Work out the finished part from the listing and answer in its coordinate system (mm). Round coordinates to 2 decimals unless told otherwise and drop trailing zeros. Order: outer loops, then holes, each group sorted by start corner. A loop starts at its lowest first (then second) coordinate and runs counter-clockwise, first axis right, second up.
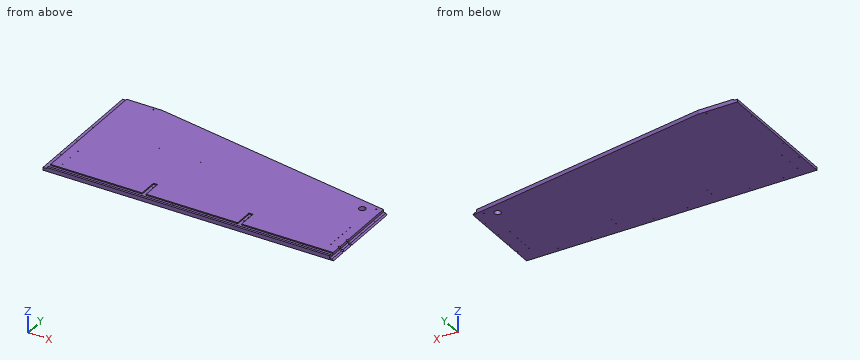
from build123d import *

# Parameters (mm, degrees)
CABSIDERIGHT_THICKNESS_DEPTH  = 17.78
LEDGECUTS_DEPTH_DEPTH         = 5.08
SKETCH9_R                     = 3.301999998
SKETCH9_R_2                   = 3.174999998
SKETCH9_R_3                   = 3.174999999
CUT_EXTRUDE4_DEPTH            = 5.08
SKETCH10_R                    = 15.08125
SKETCH10_R_2                  = 1.5875
CUT_EXTRUDE5_DEPTH            = 17.78
FRONTLEDGECUT_W               = 17.78
FRONTLEDGECUT_H               = 402.324113577
FRONTLEDGECUT_THICKNESS_DEPTH = 11.43
CUT_EXTRUDE8_DEPTH            = 594.36
SKETCH15_R                    = 2.38125
CUT_EXTRUDE9_DEPTH            = 17.78
SKETCH16_R                    = 1.5875
CUT_EXTRUDE10_DEPTH           = 12.7
SKETCH17_R                    = 4.7625
CUT_EXTRUDE11_DEPTH           = 76.2


with BuildPart() as part:
    # CabSideRight_Outline → CabSideRight_Thickness (new body)
    with BuildSketch(Plane.XY):
        Polygon((9092.234544556, -4658.6775), (10222.970833334, -4853.78125), (10222.970833334, -5253.0375), (8914.870833334, -5253.0375), (8914.870833334, -4658.6775), align=None)
    extrude(amount=-CABSIDERIGHT_THICKNESS_DEPTH)

    # CabSideRight_LedgeCuts → LedgeCuts_Depth (cut)
    with BuildSketch(Plane.XY):
        Polygon((8932.650833334, -4658.6775), (8914.870833334, -4658.6775), (8914.870833334, -5253.0375), (8932.650833334, -5253.0375), (8932.650833334, -5243.5125), (10222.970833334, -5243.5125), (10222.970833334, -5225.7325), (9792.864166668, -5225.7325), (9792.864166668, -5141.912499999), (9775.084166668, -5141.912499999), (9775.084166668, -5225.7325), (9362.757500002, -5225.7325), (9362.757500002, -5141.9125), (9344.977500002, -5141.912499999), (9344.977500002, -5225.7325), (8932.650833334, -5225.7325), align=None)
    extrude(amount=-LEDGECUTS_DEPTH_DEPTH, mode=Mode.SUBTRACT)

    # Sketch9 → Cut-Extrude4 (cut)
    with BuildSketch(Plane.XY):
        with Locations((9347.222564031, -5144.157564028)):
            Circle(SKETCH9_R)
        with Locations((9360.512435973, -5144.15756403)):
            Circle(SKETCH9_R_2)
        with Locations((9777.329230699, -5144.157564029)):
            Circle(SKETCH9_R_3)
        with Locations((9790.619102638, -5144.157564029)):
            Circle(SKETCH9_R_3)
    extrude(amount=-CUT_EXTRUDE4_DEPTH, mode=Mode.SUBTRACT)

    # Sketch10 → Cut-Extrude5 (cut)
    with BuildSketch(Plane.XY):
        with Locations((10132.081036572, -4887.549352662)):
            Circle(SKETCH10_R)
        with Locations((10165.516033334, -5148.2625)):
            Circle(SKETCH10_R_2)
        with Locations((8923.760833334, -4778.904166666)):
            Circle(SKETCH10_R_2)
        with Locations((8923.760833334, -4897.4375)):
            Circle(SKETCH10_R_2)
        with Locations((8923.760833334, -5015.970833334)):
            Circle(SKETCH10_R_2)
        with Locations((8923.760833334, -5134.504166666)):
            Circle(SKETCH10_R_2)
        with Locations((9054.570833334, -5234.6225)):
            Circle(SKETCH10_R_2)
        with Locations((9206.970833334, -5234.6225)):
            Circle(SKETCH10_R_2)
        with Locations((9353.8675, -5193.9825)):
            Circle(SKETCH10_R_2)
        with Locations((9353.8675, -5160.9625)):
            Circle(SKETCH10_R_2)
        with Locations((9486.370833334, -5234.6225)):
            Circle(SKETCH10_R_2)
        with Locations((9638.770833334, -5234.6225)):
            Circle(SKETCH10_R_2)
        with Locations((9783.974166666, -5193.9825)):
            Circle(SKETCH10_R_2)
        with Locations((9783.974166666, -5160.9625)):
            Circle(SKETCH10_R_2)
        with Locations((9918.170833334, -5234.6225)):
            Circle(SKETCH10_R_2)
        with Locations((10070.570833334, -5234.6225)):
            Circle(SKETCH10_R_2)
        with Locations((10214.080833334, -5031.58125)):
            Circle(SKETCH10_R_2)
        with Locations((10214.080833334, -4929.98125)):
            Circle(SKETCH10_R_2)
        with Locations((10165.516033334, -5091.1125)):
            Circle(SKETCH10_R_2)
        with Locations((8972.338333334, -5087.9375)):
            Circle(SKETCH10_R_2)
        with Locations((8972.338333334, -5145.0875)):
            Circle(SKETCH10_R_2)
        with Locations((8972.338333334, -5202.2375)):
            Circle(SKETCH10_R_2)
        with Locations((10165.503333334, -5176.8375)):
            Circle(SKETCH10_R_2)
        with Locations((10165.503333334, -5119.6875)):
            Circle(SKETCH10_R_2)
        with Locations((10165.503333334, -5062.5375)):
            Circle(SKETCH10_R_2)
        with Locations((10165.516033334, -5033.9625)):
            Circle(SKETCH10_R_2)
    extrude(amount=-CUT_EXTRUDE5_DEPTH, mode=Mode.SUBTRACT)

    # FrontLedgeCut → FrontLedgeCut_Thickness (cut)
    with BuildSketch(Plane.XY):
        with Locations((10214.080833334, -5051.875443212)):
            Rectangle(FRONTLEDGECUT_W, FRONTLEDGECUT_H)
    extrude(amount=-FRONTLEDGECUT_THICKNESS_DEPTH, mode=Mode.SUBTRACT)

    # FrontBevelAngleCut → Cut-Extrude8 (cut)
    with BuildSketch(Plane.XZ.offset(5253.0375)):
        Polygon((10222.970833334, -11.43), (10229.320833334, -11.43), (10222.970833334, -17.78), (10216.620833334, -11.43), align=None)
    extrude(amount=-CUT_EXTRUDE8_DEPTH, mode=Mode.SUBTRACT)

    # Sketch15 → Cut-Extrude9 (cut)
    with BuildSketch(Plane(origin=(0, 0, -17.78), x_dir=(-1, 0, 0), z_dir=(0, 0, -1))):
        with Locations((-10180.810459726, -4864.401180469)):
            Circle(SKETCH15_R)
        with Locations((-9060.71197776, -4671.132938908)):
            Circle(SKETCH15_R)
    extrude(amount=-CUT_EXTRUDE9_DEPTH, mode=Mode.SUBTRACT)

    # Sketch16 → Cut-Extrude10 (cut)
    with BuildSketch(Plane.XY):
        with Locations((9038.992342664, -4901.492108659)):
            Circle(SKETCH16_R)
        with Locations((9229.403491719, -4907.309695425)):
            Circle(SKETCH16_R)
        with Locations((9419.814640773, -4913.127282192)):
            Circle(SKETCH16_R)
    extrude(amount=-CUT_EXTRUDE10_DEPTH, mode=Mode.SUBTRACT)

    # Sketch17 → Cut-Extrude11 (cut)
    with BuildSketch(Plane(origin=(5086.511865443, 0, -5086.511865443), x_dir=(0.707106781, 0, 0.707106781), z_dir=(-0.707106781, 0, 0.707106781))):
        with Locations((7216.159641553, -5119.6875)):
            Circle(SKETCH17_R)
        with Locations((7216.159641553, -5176.8375)):
            Circle(SKETCH17_R)
    extrude(amount=-CUT_EXTRUDE11_DEPTH, mode=Mode.SUBTRACT)


solid = part.part
Item 1: Find the intervals of material crossed by line 1 along X through (y, z) = (-4996.5, -11); line 2 along X through (y, z) = (-4915, -2.5); line 3 along Y through (x, z) = (9837, -4), in increasing order.
Item 2: Find section C-C (x = 9750.5). Write down the section's boundary in (y, z).
Item 3: Find section A-A (x = 9277). Write down the section's boundary in (y, z), plus the area to 3 significant figures.
Item 4: Find section B-B (y = -4702). Write down the section's boundary in (x, z), plus the area to 3 significant figures.
Item 5: Given pin 1 (5 mm diameter, centred on x = 9054.57, y = -5234.62, fed in from +Z); pin 2 (1 mm diameter, centred on x = 9419, y = -4913.5, fed in from +Z); pin 3 (3 mm diameter, centred on x = 8923.76, y = -5134.5, fed in from +Z); pin 4 (2 mm diameter, centred on x = 9388.5, z = -6, fed in from +Y), each flat-ended and moving along its own axis, determine where each tip first touches the part or whether it passes through.
Model answer:
1. line 1: x = 8914.87 to 10205.19
1. line 2: x = 8932.65 to 10205.19
1. line 3: y = -5253.04 to -5243.51, -5225.73 to -4787.18
2. outline: (-5253.04, -17.78) - (-4772.26, -17.78) - (-4772.26, 0) - (-5225.73, 0) - (-5225.73, -5.08) - (-5243.51, -5.08) - (-5243.51, 0) - (-5253.04, 0) - close
3. outline: (-5253.04, -17.78) - (-4690.56, -17.78) - (-4690.56, 0) - (-5225.73, 0) - (-5225.73, -5.08) - (-5243.51, -5.08) - (-5243.51, 0) - (-5253.04, 0) - close
3. area: 9,910 mm2
4. outline: (8914.87, -17.78) - (9343.31, -17.78) - (9343.31, 0) - (8932.65, 0) - (8932.65, -5.08) - (8914.87, -5.08) - close
4. area: 7,530 mm2
5. pin 1: stops at z = -5.08
5. pin 2: stops at z = -12.7
5. pin 3: passes through
5. pin 4: stops at y = -4709.62
